Build history of the part. All positions in model axes, mm. A direction names the side the tool comes from. Give positions to 0.01 mm unless a question says otherwise; leave off trailing zeros. Order: outer loops, then holes, each group sorted by start corner. A loop starts at its lowest first (then second) coordinate and runs counter-clockwise, first axis right, second up. Notation, with made-up numbers: (-5, 47.25) - (46, 47.25) arc R19 cw to (46, 65.25) - close; hole circle Ø2 at (8.5, -40). An arc over 180 degrees is marked (long way). One line per item, written item: value.
```python
from build123d import *

# Parameters (mm, degrees)
F0_R     = 1
F1_DEPTH = 13
F3_DEPTH = 2.5
F4_R     = 1.5
F5_R     = 0.5
F6_SIZE2 = 0.8660254038
F6_SIZE  = 1.5


with BuildPart() as f1:
    # F0 (on Front) → F1 (new body)
    with BuildSketch(Plane.XZ):
        Polygon((0, 25), (0, 0), (8, 0), (8, 11), (13, 11), (13, 25), align=None)
        with Locations((5.5, 2.6)):
            Circle(F0_R, mode=Mode.SUBTRACT)
        with Locations((5.5, 11)):
            Circle(F0_R, mode=Mode.SUBTRACT)
        with Locations((6.5, 21.5)):
            Circle(F0_R, mode=Mode.SUBTRACT)
    extrude(amount=F1_DEPTH)

    # F2 (on face) → F3 (cut)
    with BuildSketch(Plane.YZ.offset(8)):
        with BuildLine():
            Line((-13, 5.1547005384), (-11, 4))
            Line((-11, 4), (-10.3, 4))
            ThreePointArc((-10.3, 4), (-7.8, 6.5), (-10.3, 9))
            Line((-10.3, 9), (-11, 9))
            Line((-11, 9), (-13, 7.8452994616))
            Line((-13, 7.8452994616), (-13, 5.1547005384))
        make_face()
    extrude(amount=-F3_DEPTH, mode=Mode.SUBTRACT)

    # F4
    f4_edges = [f1.edges().sort_by_distance(p)[0] for p in [
        (8, -6.5, 0),
        (0, -6.5, 0),
        (13, -6.5, 11),
    ]]
    fillet(f4_edges, radius=F4_R)

    # F5
    f5_edges = [f1.edges().sort_by_distance(p)[0] for p in [
        (8, -6.5, 11),
    ]]
    fillet(f5_edges, radius=F5_R)

    # F6
    f6_edges = [f1.edges().sort_by_distance(p)[0] for p in [
        (13, 0, 18.75),
    ]]
    f6_side = f1.faces().sort_by_distance((13, -6.5, 18.75))[0]
    chamfer(f6_edges, length=F6_SIZE, length2=F6_SIZE2, reference=f6_side)


solid = f1.part
```
(1) Slice it at C-C, the plane z = 6.5. Give the cut face in (x, y), and give its area (3 significant figures).
Completed:
outline: (0, -13) - (5.5, -13) - (5.5, -7.8) - (8, -7.8) - (8, -1.5) - (7.13, 0) - (0.87, 0) - (0, -1.5) - close
area: 89.7 mm²
(2) Pin check, flat tips, straight feed: P1, Ø4, axis at y = -9.5, z = 5.5, coming from the +X side; P2, Ø1.8, axis at x = 5.5, z = 2.6, coming from the -Y side; P3, Ø3.5, axis at x = 10, y = -10, coming from the -Z side; P4, Ø2.5, axis at x = 5.5, z = 11, coming from the +Y side. Stop position of each tip, or through.
Completed:
P1: x = 8
P2: through
P3: z = 10.93
P4: y = 0
(3) 3-axis set-ups, long thin cutter, end or side, ignore diameter. For faces 1 (the face through (0.43, -7.33, 0.45)), 2 (the face through (6.8, -7.8, 6.4)), 3 (the face through (10, -7, 11)), 4 (the face through (9.98, -0.74, 11.44)), 5 (the face through (6.283, -6.409, 20.524)): which of +Z, -Z, +X, -X, +Y, -Y reach the whole face in a straight line?
Completed:
face 1: -Z, -X, +Y, -Y
face 2: +X
face 3: -Z, +X, +Y, -Y
face 4: -Z, +X, +Y
face 5: +Y, -Y
(4) Slice it at B-B, the plane y = -4. Give the cut face in (x, z).
Completed:
outline: (0, 1.5) arc R1.5 ccw to (1.5, 0) - (6.5, 0) arc R1.5 ccw to (8, 1.5) - (8, 10.5) arc R0.5 cw to (8.5, 11) - (11.5, 11) arc R1.5 ccw to (13, 12.5) - (13, 25) - (0, 25) - close; hole circle Ø2 at (5.5, 2.6); hole circle Ø2 at (5.5, 11); hole circle Ø2 at (6.5, 21.5)
(5) Slice it at D-D, the plane z = 2.6. Give the cut face in (x, y), and give its area (3 significant figures).
Completed:
outline: (0, -13) - (4.5, -13) - (4.5, 0) - (0.87, 0) - (0, -1.5) - close; (6.5, -13) - (8, -13) - (8, -1.5) - (7.13, 0) - (6.5, 0) - close
area: 76.7 mm²
(6) Slice it at A-A, the plane z = 21. Give the cut face in (x, y), and give its area (3 significant figures).
Completed:
outline: (0, -13) - (5.63, -13) - (5.63, 0) - (0.87, 0) - (0, -1.5) - close; (7.37, -13) - (13, -13) - (13, -1.5) - (12.13, 0) - (7.37, 0) - close
area: 145 mm²
(7) Pull direction X, two halves, no side cores. Call faces 6 (the face through (12.24, -0.74, 11.74)), 7 (the face through (5, -13, 13)), 8 (the face through (4.7, -6.4, 10.4)): +X half, -X half, draft (parallel to the pull), parting line (faces both ways), or undercut.
Completed:
face 6: +X half
face 7: draft
face 8: undercut
(8) Drill centre lines: line 1 (X direction, y = -1.75, z = 3.5); line 2 (X direction, y = -10, z = 22); line 3 (Z direction, x = 8.5, y = -11). Where is each one in solid material? Low to high.
Completed:
line 1: 0 to 5.06, 5.94 to 8
line 2: 0 to 5.63, 7.37 to 13
line 3: 11 to 25
